Input: dimensioned drawing with shaded views. Units: mm. Origin: part minimum x, y, z. Give positions to 0.01 mm unless a question says otherwise; leave off trailing zeros. Write each loop counter-clockwise with the first axis right and the second up, starting at its lowest first coordinate (ties: lowest second). Pieces come first, ordered by that corner, then holes.
Q1. Section A-A (x = 119.5). Return the cut outline in (y, z) (1 decimal).
Q2. Section C-C (x = 102). Return the cut outline in (y, z), plus the area to 3 significant figures.
Q3. Line query: line 1 (Z direction, x = 119, y = 0.25) (1 decimal); line 2 (X direction, y = 1.05, z = 5.5); line 3 (Z direction, x = 106, y = 0.2). Output: solid intervals per line, ascending.
Q4. Section B-B (y = 0.9). State how many separate pieces and enclosed holes the cut face has, plus the area to 3 significant figures.
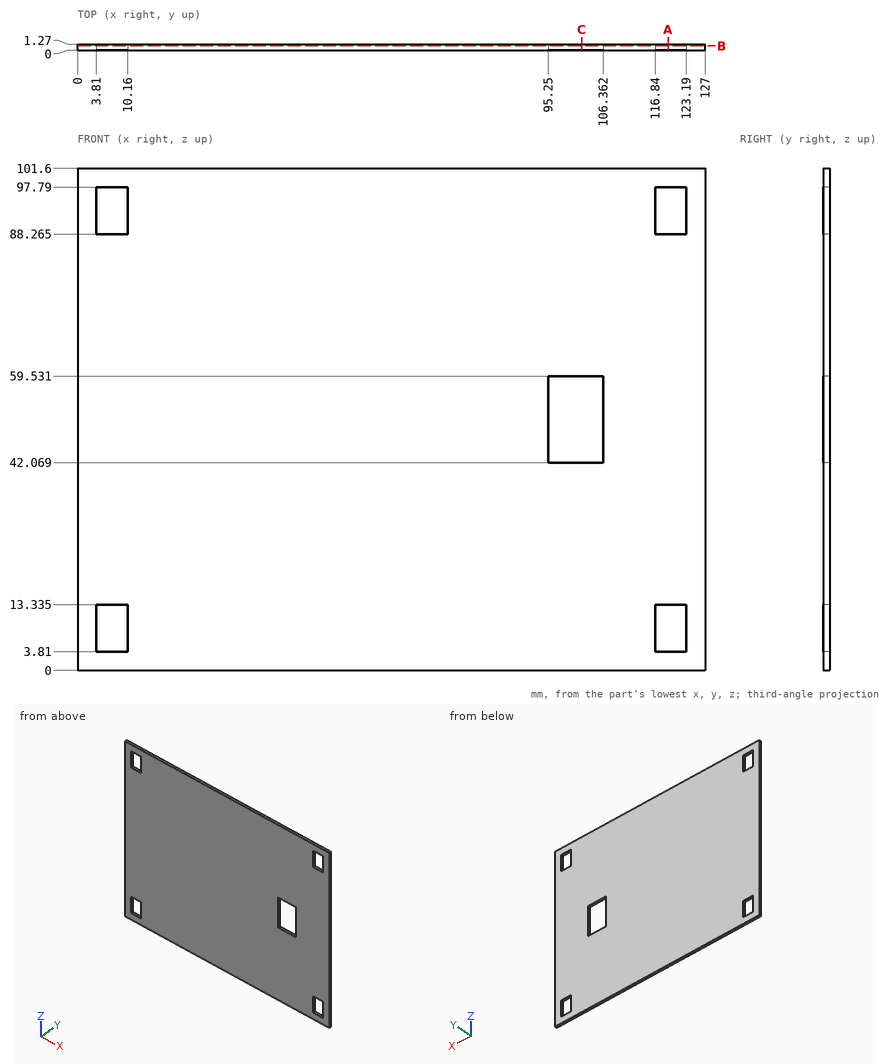
Computed:
1. outline: (0, 0) - (1.3, 0) - (1.3, 3.8) - (0, 3.8) - close; (0, 13.3) - (1.3, 13.3) - (1.3, 88.3) - (0, 88.3) - close; (0, 97.8) - (1.3, 97.8) - (1.3, 101.6) - (0, 101.6) - close
2. outline: (0, 0) - (1.27, 0) - (1.27, 42.07) - (0, 42.07) - close; (0, 59.53) - (1.27, 59.53) - (1.27, 101.6) - (0, 101.6) - close
2. area: 107 mm2
3. line 1: z = 0 to 3.8, 13.3 to 88.3, 97.8 to 101.6
3. line 2: x = 0 to 3.81, 10.16 to 116.84, 123.19 to 127
3. line 3: z = 0 to 42.07, 59.53 to 101.6
4. separate pieces: 1
4. enclosed holes: 5
4. area: 12,500 mm2
